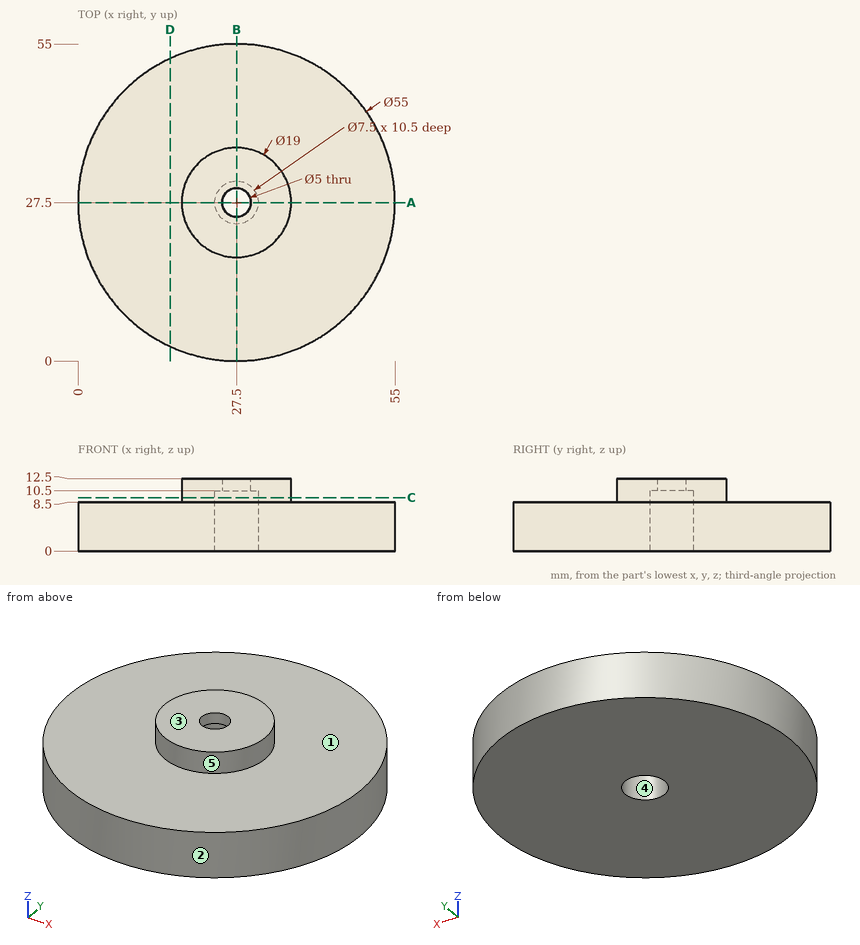
Check sheet for the drawn part. Datum: minimum x, y, z corner. Units: mm. A direction names the side the tool comes from. Give positions to 0.01 mm unless a question says otherwise; leave off trailing zeros. Write each loop counter-clockwise with the first axis right and the second up, starting at its lowest first coordinate (ties: lowest second). Pieces come first, ordered by that corner, then holes. Notation, with made-up numbers: M 67,-20.75 L 115,-20.75 A5 cw 115,-15.75 Z; hole C -7.5,-17.75 d5. An arc over 180 degrees is marked long. Write item = value, one per line.
(1) Go/stop test with flat-tipped pins: pin 1 Ø5 at (x, y) = (33, 17.5) entering from +Z; pin 2 Ø3 at (x, z) = (33.5, 1.5) entering from -Y; pin 3 Ø3 at (x, y) = (27.5, 27.5) entering from -Z; pin 4 Ø6 at (x, z) = (38, 10.5) entering from -Y. Record where each tip stops, or that it passes through.
Found:
pin_1 = 12.5
pin_2 = 0.37
pin_3 = through
pin_4 = 1.27
(2) Draft check along X on the marked faces 3, 4 and 5. Enter one of: released by +X, released by -X, zero draft, split by the parting line, or undercut.
Found:
face_3 = zero draft
face_4 = undercut
face_5 = split by the parting line
(3) Material ranges on line 1 (Y direction, x = 27.5, z = 3.5); line 2 (Y direction, x = 27.5, z = 12); line 3 (Z direction, x = 8.5, y = 24), recorded low to high.
Found:
line_1 = 0 to 23.75, 31.25 to 55
line_2 = 18 to 25, 30 to 37
line_3 = 0 to 8.5
(4) Sectioned sample at C-C (z = 9.25). Record the cut outline in (x, y).
Found:
outline = C 27.5,27.5 d19; hole C 27.5,27.5 d7.5
(5) Sectioned sample at A-A (y = 27.5). Record the cut outline in (x, z).
Found:
outline = M 0,0 L 23.75,0 L 23.75,10.5 L 25,10.5 L 25,12.5 L 18,12.5 L 18,8.5 L 0,8.5 Z; M 30,10.5 L 31.25,10.5 L 31.25,0 L 55,0 L 55,8.5 L 37,8.5 L 37,12.5 L 30,12.5 Z
(6) Sectioned sample at D-D (x = 16). Record the cut outline in (y, z), then the cut area to 3 significant figures.
Found:
outline = M 2.52,0 L 52.48,0 L 52.48,8.5 L 2.52,8.5 Z
area = 425 mm2
(7) Access from +Z, -Z, +X, -X, +Y, -Y to the whole of each face (thin tool, end or side, straight path). Record for the marked faces 1 and 2.
Found:
face_1 = +Z
face_2 = +Z, -Z
